Can you work these out from the drawing? Everything is in mm from the part's minimum corner. A direction names the side the tool comes from. Round coordinates to 2 decimals unless told otherwise and drop trailing zeros. Order: outer loops, then holes, each group sorted by start corner. A loop starts at its lowest first (then second) coordinate and runs counter-clockwise, first axis right, second up. Notation, with made-up numbers: M -22,19.5 L 11,19.5 A32 ccw 11,46.5 Z; hole C 82,60.5 d8. An arc over 180 degrees is marked long. Write item = value, one per line. Start each with the question number.
Item 1: I want a section at A-A, the plane y = 6. List the corners of the cut face in (x, z) for me.
Item 2: For the marked faces 5, 6, 7, 8 and 9, which set-ups out of +Z, -Z, +X, -X, +Y, -Y let a thin tool reach every point of the face, with its end or its side?
Item 3: I want a section at D-D, the plane z = 23.75. List the corners of the cut face in (x, y) for me.
Item 4: I'm going to push flat-ended pins straight in: P1, Ø3, axis at x = 2, y = 6.5, coming from the -Z side; P2, Ø2.5, axis at y = 4, z = 24.5, coming from the -X side; P3, Ø1.5, axis at x = 4, z = 24, coming from the +Y side. Where does each tip first touch, or does it pass through?
Item 5: We'd pull the mould along Y, two halves only. Please class the marked faces 1, 2, 3 and 4: pulls with the +Y half, pulls with the -Y half, needs draft (parallel to the pull), parting line crosses it, or undercut.
Item 6: I want a section at B-B, the plane x = 6. List the corners of the cut face in (y, z) for me.
Item 7: Please list where these lines run through material, in increasing order: L1, parallel to Y at x = 4.25, z = 12; L2, parallel to X at y = 1.05, z = 6; L3, parallel to Z at x = 3.5, y = 3.25.
Item 8: I want a section at C-C, the plane y = 2. List the corners of the cut face in (x, z) for me.
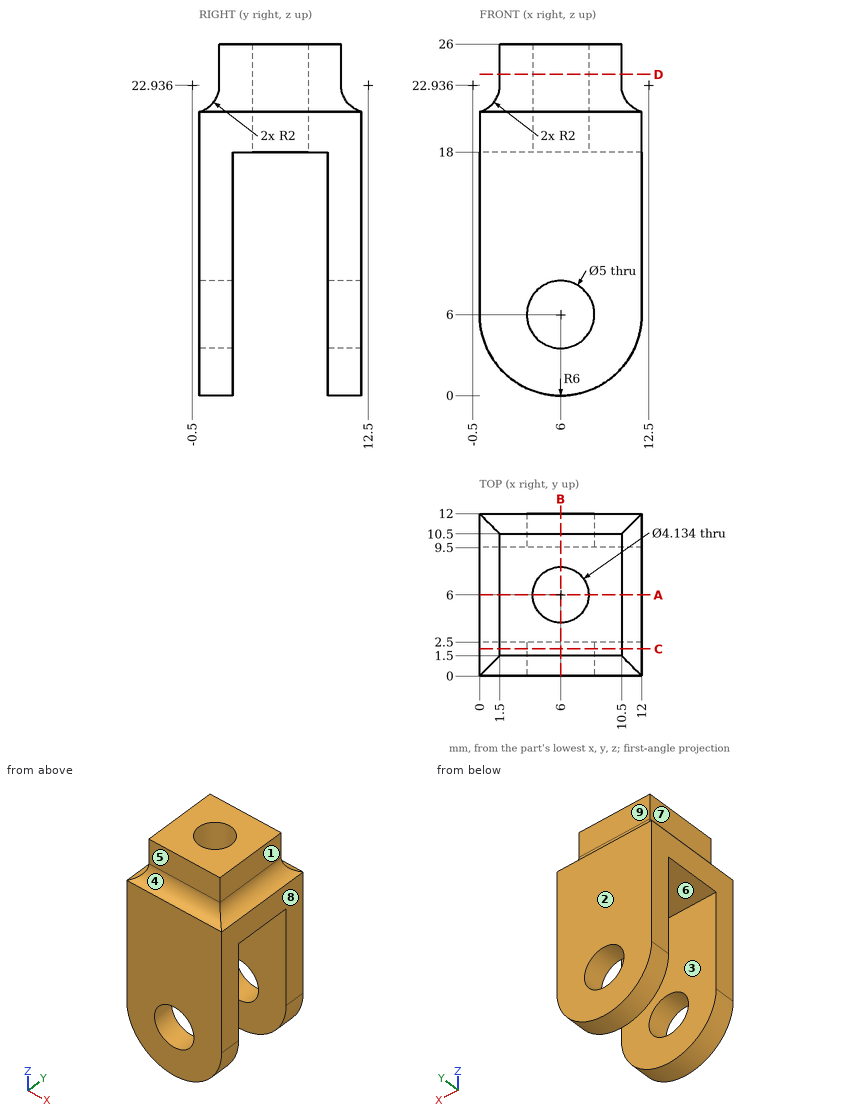
Filled in:
q1.outline = M 0,18 L 3.93,18 L 3.93,26 L 1.5,26 L 1.5,22.94 A2 cw 0,21 Z; M 8.07,18 L 12,18 L 12,21 A2 cw 10.5,22.94 L 10.5,26 L 8.07,26 Z
q2.face_5 = +Z, +X, -X, -Y
q2.face_6 = -Z, +X, -X
q2.face_7 = +Z, -X, +Y, -Y
q2.face_8 = +Z, -Z, +X, +Y, -Y
q2.face_9 = +Z, +X, -X, +Y
q3.outline = M 1.5,1.5 L 10.5,1.5 L 10.5,10.5 L 1.5,10.5 Z; hole C 6,6 d4.13
q4.P1 = 18
q4.P2 = 1.5
q4.P3 = 10.5
q5.face_1 = needs draft
q5.face_2 = pulls with the +Y half
q5.face_3 = undercut
q5.face_4 = pulls with the -Y half
q6.outline = M 0,0 L 2.5,0 L 2.5,3.5 L 0,3.5 Z; M 0,8.5 L 2.5,8.5 L 2.5,18 L 3.93,18 L 3.93,26 L 1.5,26 L 1.5,22.94 A2 cw 0,21 Z; M 8.07,18 L 9.5,18 L 9.5,8.5 L 12,8.5 L 12,21 A2 cw 10.5,22.94 L 10.5,26 L 8.07,26 Z; M 9.5,0 L 12,0 L 12,3.5 L 9.5,3.5 Z
q7.L1 = 0 to 2.5, 9.5 to 12
q7.L2 = 0 to 3.5, 8.5 to 12
q7.L3 = 18 to 26
q8.outline = M 0,6 A6 ccw 12,6 L 12,21 A2 cw 10.5,22.94 L 10.5,26 L 1.5,26 L 1.5,22.94 A2 cw 0,21 Z; hole C 6,6 d5
